from build123d import *

# Parameters (mm, degrees)
PAD_DEPTH       = 3.175
SKETCH001_R     = 1.5875
POCKET_DEPTH    = 3.176
SKETCH002_R     = 1.5
POCKET001_DEPTH = 3.176
SKETCH003_R     = 1.1684
POCKET002_DEPTH = 3.176


with BuildPart() as part:
    # Sketch → Pad (new body)
    with BuildSketch(Plane.XY):
        with BuildLine():
            ThreePointArc((-55.372, 105.283), (-67.944359, 100.075359), (-73.152, 87.503))
            Line((-73.152, -87.503), (-73.152, 87.503))
            ThreePointArc((-73.152, -87.503), (-67.944359, -100.075359), (-55.372, -105.283))
            Line((55.372, -105.283), (-55.372, -105.283))
            ThreePointArc((55.372, -105.283), (67.944359, -100.075359), (73.152, -87.503))
            Line((73.152, 87.503), (73.152, -87.503))
            ThreePointArc((73.152, 87.503), (67.944359, 100.075359), (55.372, 105.283))
            Line((-55.372, 105.283), (55.372, 105.283))
        make_face()
    extrude(amount=PAD_DEPTH)

    # Sketch001 (on DatumPlane) → Pocket (cut, through all)
    with BuildSketch(Plane.XY.offset(3.175)):
        with Locations((-65.024, 96.774)):
            Circle(SKETCH001_R)
        with Locations((65.024, 96.774)):
            Circle(SKETCH001_R)
        with Locations((65.024, -96.774)):
            Circle(SKETCH001_R)
        with Locations((-65.024, -96.774)):
            Circle(SKETCH001_R)
        with Locations((-66.929, 0)):
            Circle(SKETCH001_R)
        with Locations((66.929, 0)):
            Circle(SKETCH001_R)
    extrude(amount=-POCKET_DEPTH, mode=Mode.SUBTRACT)

    # Sketch002 (on DatumPlane) → Pocket001 (cut, through all)
    with BuildSketch(Plane.XY.offset(3.175)):
        with Locations((-38.1, 25.905)):
            Circle(SKETCH002_R)
        with Locations((38.1, 25.905)):
            Circle(SKETCH002_R)
        with Locations((-20.828, -25.905)):
            Circle(SKETCH002_R)
        with Locations((20.828, -25.905)):
            Circle(SKETCH002_R)
        with BuildLine():
            Line((-18.288, -29.08), (-18.288, -40.51))
            ThreePointArc((-18.288, -40.51), (-17.916026, -41.408026), (-17.018, -41.78))
            Line((-17.018, -41.78), (17.018, -41.78))
            ThreePointArc((17.018, -41.78), (17.916026, -41.408026), (18.288, -40.51))
            Line((18.288, -40.51), (18.288, -29.08))
            Line((18.288, -29.08), (18.288, -24.635))
            ThreePointArc((19.558, -23.365), (18.659974, -23.736974), (18.288, -24.635))
            Line((19.558, -23.365), (46.99, -23.365))
            ThreePointArc((46.99, -23.365), (47.888026, -22.993026), (48.26, -22.095))
            Line((48.26, -22.095), (48.26, 22.095))
            ThreePointArc((48.26, 22.095), (47.888026, 22.993026), (46.99, 23.365))
            Line((46.99, 23.365), (36.83, 23.365))
            ThreePointArc((35.56, 24.635), (35.931974, 23.736974), (36.83, 23.365))
            Line((35.56, 24.635), (35.56, 29.08))
            Line((35.56, 29.08), (35.56, 91.31))
            ThreePointArc((35.56, 91.31), (35.188026, 92.208026), (34.29, 92.58))
            Line((34.29, 92.58), (-34.29, 92.58))
            ThreePointArc((-34.29, 92.58), (-35.188026, 92.208026), (-35.56, 91.31))
            Line((-35.56, 91.31), (-35.56, 29.08))
            Line((-35.56, 29.08), (-35.56, 24.635))
            ThreePointArc((-36.83, 23.365), (-35.931974, 23.736974), (-35.56, 24.635))
            Line((-36.83, 23.365), (-46.99, 23.365))
            ThreePointArc((-46.99, 23.365), (-47.888026, 22.993026), (-48.26, 22.095))
            Line((-48.26, 22.095), (-48.26, -22.095))
            ThreePointArc((-48.26, -22.095), (-47.888026, -22.993026), (-46.99, -23.365))
            Line((-46.99, -23.365), (-19.558, -23.365))
            ThreePointArc((-18.288, -24.635), (-18.659974, -23.736974), (-19.558, -23.365))
            Line((-18.288, -24.635), (-18.288, -29.08))
        make_face()
    extrude(amount=-POCKET001_DEPTH, mode=Mode.SUBTRACT)

    # Sketch003 (on DatumPlane) → Pocket002 (cut, through all)
    with BuildSketch(Plane.XY.offset(3.175)):
        with Locations((-57.15, 88.9)):
            Circle(SKETCH003_R)
        with Locations((57.15, 88.9)):
            Circle(SKETCH003_R)
        with Locations((57.15, 0)):
            Circle(SKETCH003_R)
        with Locations((57.15, -88.9)):
            Circle(SKETCH003_R)
        with Locations((-57.15, -88.9)):
            Circle(SKETCH003_R)
        with Locations((-57.15, 0)):
            Circle(SKETCH003_R)
    extrude(amount=-POCKET002_DEPTH, mode=Mode.SUBTRACT)


solid = part.part
The listing builds one solid part. Answer for the finished solid, in the listing's coordinates (mm). Coordinates: 2 decimals unless noted, no trailing zeros. Write each loop counter-clockwise with the first axis right and the second up, starting at its lowest first coordinate (ties: lowest second). Pieces come first, ordered by that corner, then holes. Notation, with made-up numbers: M 13.25,-22.75 L 18.25,-22.75 A33 cw 18.25,10.25 Z; hole C -10.5,13 d10. An arc over 180 degrees is marked long. Use one line per item in the form item = value.
Item 1: Find section C-C, the plane z = 0.6. Give the number of separate pieces and of enclosed holes in the cut face, plus the area to 3 significant figures.
Model answer:
separate_pieces = 1
enclosed_holes = 17
area = 20,300 mm2
Item 2: Find the intervals of material crossed by probe 1 along Y at (x, z) = (-38.1, 1.3) (3 decimals); probe 2 along Y at (x, z) = (47, 2.95); probe 3 along X at (y, z) = (37, 0.7), in increasing order.
Model answer:
probe_1 = -105.283 to -23.365, 23.365 to 24.405, 27.405 to 105.283
probe_2 = -105.28 to -23.36, 23.36 to 105.28
probe_3 = -73.15 to -35.56, 35.56 to 73.15
Item 3: Find section B-B, the plane y = 77. Give the vertices of the cut face in (x, z) (3 decimals).
Model answer:
outline = M -73.152,0 L -35.56,0 L -35.56,3.175 L -73.152,3.175 Z; M 35.56,0 L 73.152,0 L 73.152,3.175 L 35.56,3.175 Z
Item 4: Find section A-A, the plane x = 7.5. Give the vertices of the cut face in (y, z) (3 decimals), plus the area to 3 significant figures.
Model answer:
outline = M -105.283,0 L -41.78,0 L -41.78,3.175 L -105.283,3.175 Z; M 92.58,0 L 105.283,0 L 105.283,3.175 L 92.58,3.175 Z
area = 242 mm2
